Here's how the part is built. I have some questions about the finished solid (model axes, mm). Face numbers are marked on the shaded views. A direction names the side the tool comes from. Coordinates: 2 decimals unless noted, no trailing zeros. Write each loop counter-clockwise with the first axis right and the second up, starting at its lowest first coordinate (ties: lowest second). Pieces come first, ordered by that corner, then holes. Notation, with made-up numbers: (42, 71.25) -> (68, 71.25) arc R34 cw to (68, 110.25) -> close; hole circle Ø6 at (51, 10.5). An arc over 180 degrees is marked (long way). Put each result on its own line as item: value.
```python
from build123d import *

# Parameters (mm, degrees)
ESBO_O1_W               = 92
ESBO_O1_H               = 12.7
FLANGE_BASE1_DEPTH      = 3.18
DOBRA_START             = -6.35
DOBRA_ESBO_ADA1_DEPTH   = 12.7
DOBRA_ESBO_ADA1_2_DEPTH = 12.7
ESBO_O8_R               = 2.75
CORTE_EXTRUS_O1_DEPTH   = 10
ESBO_O10_R              = 2.25
CORTE_EXTRUS_O3_DEPTH   = 10


# Read off the part's stored shape, not the designer's step: Dobra esboçada1
# Sheet-metal steps are written as plain solids
with BuildPart() as part:
    # Esboço1 → Flange-base1 (new body)
    with BuildSketch(Plane.XY):
        Rectangle(ESBO_O1_W, ESBO_O1_H)
    extrude(amount=-FLANGE_BASE1_DEPTH)

    # Dobra esboçada1 outline → Dobra esboçada1 (cut)
    with BuildSketch(Plane(origin=(0, 0, 0), x_dir=(1, 0, 0), z_dir=(0, 1, 0)).offset(DOBRA_START)):
        with BuildLine():
            ThreePointArc((15.50243384, 3.18), (18.68243384, 2.327921568), (21.010355408, 0))
            Line((21.010355408, 0), (46, 0))
            Line((46, 0), (46, 3.18))
            Line((46, 3.18), (15.50243384, 3.18))
        make_face()
    extrude(amount=DOBRA_ESBO_ADA1_DEPTH, mode=Mode.SUBTRACT)

    # Dobra esbo_ada1 2 outline → Dobra esbo_ada1 2 (add)
    with BuildSketch(Plane(origin=(0, 0, 0), x_dir=(1, 0, 0), z_dir=(0, 1, 0)).offset(DOBRA_START)):
        with BuildLine():
            Line((18.256394624, -1.59), (31.007611545, -23.675755564))
            Line((31.007611545, -23.675755564), (33.761572329, -22.085755564))
            Line((33.761572329, -22.085755564), (21.010355408, 0))
            Line((21.010355408, 0), (15.50243384, 0))
            ThreePointArc((15.50243384, 0), (17.09243384, -0.426039216), (18.256394624, -1.59))
        make_face()
    extrude(amount=DOBRA_ESBO_ADA1_2_DEPTH)

    # Esboço8 → Corte-extrusão1 (cut)
    with BuildSketch(Plane(origin=(0, 0, -3.18), x_dir=(-1, 0, 0), z_dir=(0, 0, -1))):
        with Locations((21.455259123, 0)):
            Circle(ESBO_O8_R)
    extrude(amount=-CORTE_EXTRUS_O1_DEPTH, mode=Mode.SUBTRACT)

    # Esboço10 → Corte-extrusão3 (cut)
    with BuildSketch(Plane(origin=(15.757766556, 0, -9.097750763), x_dir=(-0.49999999999999806, 0, -0.8660254037844398), z_dir=(0.8660254037844397, 0, -0.499999999999998))):
        with Locations((-29.427611545, 0.33)):
            Circle(ESBO_O10_R)
    extrude(amount=-CORTE_EXTRUS_O3_DEPTH, mode=Mode.SUBTRACT)


solid = part.part
```
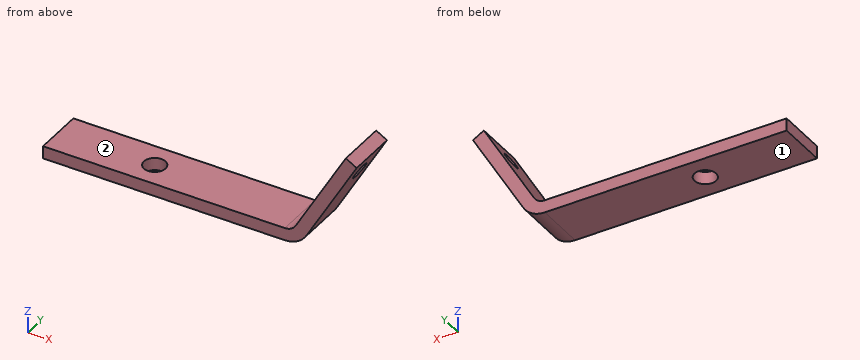
Item 1: Imagine slicing it at C-C on z = 4.5. Write out the boundary of the cut face in (x, y), then the cut area to 3 significant figures.
Output:
outline: (19.94, -6.35) -> (23.61, -6.35) -> (23.61, 6.35) -> (19.94, 6.35) -> close
area: 46.6 mm²
Item 2: Which directions (+Z, -Z, +X, -X, +Y, -Y) give clear straight access to the entire face, cutting with the end or side of a thin tool? Please do the marked faces 1 and 2.
Output:
face 1: -Z, +X, -X, +Y, -Y
face 2: +Z, -X, +Y, -Y
Item 3: Imagine slicing it at A-A on x = -22. Write out the boundary of the cut face in (y, z), then the cut area to 3 significant figures.
Output:
outline: (-6.35, -3.18) -> (-2.7, -3.18) -> (-2.7, 0) -> (-6.35, 0) -> close; (2.7, -3.18) -> (6.35, -3.18) -> (6.35, 0) -> (2.7, 0) -> close
area: 23.2 mm²
Item 4: For P1, Ø4, axis at x = 22.5, y = 1.5, coming from the -Z side; P2, Ø6.5, axis at x = -21.46, y = 0, coming from the +Z side; P3, Ø12, axis at x = 15.5, z = 14, coming from the -Y side, each with a flat end and sliding along its axis, tell me the tip position at first contact or that it passes through.
Output:
P1: stops at z = -0.75
P2: stops at z = 0
P3: passes through
Item 5: Imagine slicing it at D-D on x = 5. Write out the boundary of the cut face in (y, z), then the cut area to 3 significant figures.
Output:
outline: (-6.35, -3.18) -> (6.35, -3.18) -> (6.35, 0) -> (-6.35, 0) -> close
area: 40.4 mm²
Item 6: Imagine slicing it at B-B on y = -4.25. Write out the boundary of the cut face in (x, z), then the cut area to 3 significant figures.
Output:
outline: (-46, -3.18) -> (15.5, -3.18) arc R6.36 ccw to (21.01, 0) -> (33.76, 22.09) -> (31.01, 23.68) -> (18.26, 1.59) arc R3.18 cw to (15.5, 0) -> (-46, 0) -> close
area: 293 mm²
Item 7: Please list where these lines run through material, in increasing order: line 1 along Z through (x, y) = (-2.5, -5); line 2 along X through (y, z) = (0.75, 8); line 3 along X through (y, z) = (4.5, 19.5). Write a range as from..to.
Output:
line 1: z = -3.18..0
line 2: x = 21.96..25.63
line 3: x = 28.6..32.27
